Design review of the part built by this model. Coordinates are the model's own, in mm. Face numbers are marked on the shaded views. Give positions to 0.01 mm unless a question says otherwise; leave off trailing zeros. Loops run counter-clockwise (first coordinate to the right, second up) from the corner with the lowest first, then second, coordinate; pieces in that order, holes last. Notation, with made-up numbers: (17.5, -35.75) - (57.5, -35.75) arc R20 cw to (57.5, -20.75) - close; hole circle Ø8 at (-5, 74.25). An arc over 180 degrees is marked (long way). Write each question's results on one line, items separated by ' | '.
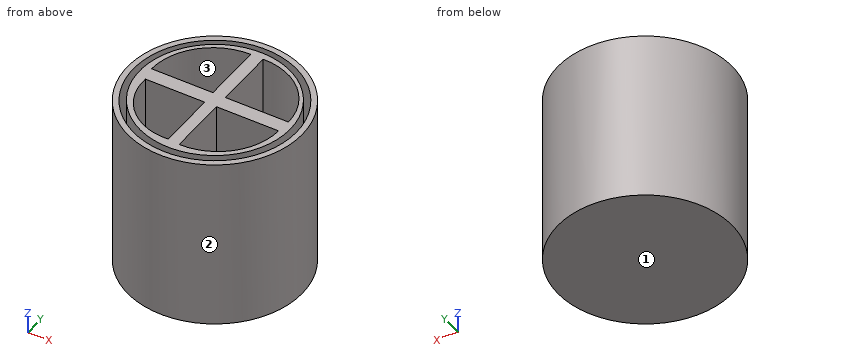
```python
from build123d import *

# Parameters (mm, degrees)
F0_R     = 38.567191
F1_DEPTH = 76.708
F2_T     = -2.54
F3_R     = 33.240041
F4_DEPTH = 74.422
F6_DEPTH = 75.946


with BuildPart() as f1:
    # F0 (on Top) → F1 (new body)
    with BuildSketch(Plane.XY):
        Circle(F0_R)
    extrude(amount=F1_DEPTH)

    # F2
    f2_openings = [f1.faces().sort_by_distance(p)[0] for p in [
        (0, 0, 76.708),
    ]]
    offset(amount=F2_T, openings=f2_openings)

    # F3 (on face) → F4 (join)
    with BuildSketch(Plane.XY.offset(2.54)):
        Circle(F3_R)
    extrude(amount=F4_DEPTH)

    # F5 (on face) → F6 (cut)
    with BuildSketch(Plane.XY.offset(76.962)):
        with BuildLine():
            ThreePointArc((30.418547, 3.318387), (22.14181, 22.611564), (2.580967, 30.234193))
            Line((2.580967, 30.234193), (2.580967, 3.318387))
            Line((2.580967, 3.318387), (30.418547, 3.318387))
        make_face()
        with BuildLine():
            Line((30.049838, -3.134032), (2.580967, -3.134032))
            Line((2.580967, -3.134032), (2.580967, -29.681129))
            ThreePointArc((2.580967, -29.681129), (21.794231, -22.076646), (30.049838, -3.134032))
        make_face()
        with BuildLine():
            Line((-2.949678, 3.318387), (-2.949678, 30.234193))
            ThreePointArc((-2.949678, 30.234193), (-22.011865, 22.326152), (-30.049838, 3.318387))
            Line((-30.049838, 3.318387), (-2.949678, 3.318387))
        make_face()
        with BuildLine():
            Line((-2.580968, -29.128065), (-2.580968, -3.134032))
            Line((-2.580968, -3.134032), (-28.759355, -3.134032))
            ThreePointArc((-28.759355, -3.134032), (-21.580145, -22.082946), (-2.580968, -29.128065))
        make_face()
    extrude(amount=-F6_DEPTH, mode=Mode.SUBTRACT)


solid = f1.part
```
Item 1: We need section D-D on y = -9. Give the boundary of the cut face in (x, z).
Output values:
outline: (-37.5, 0) - (37.5, 0) - (37.5, 76.71) - (34.88, 76.71) - (34.88, 2.54) - (32, 2.54) - (32, 76.96) - (29.29, 76.96) - (29.29, 1.02) - (2.58, 1.02) - (2.58, 76.96) - (-2.58, 76.96) - (-2.58, 1.02) - (-28.43, 1.02) - (-28.43, 76.96) - (-32, 76.96) - (-32, 2.54) - (-34.88, 2.54) - (-34.88, 76.71) - (-37.5, 76.71) - close
Item 2: Wall thickness on probe 1 along Y at (x, z) = (0, 34.5); probe 2 along Y at (x, z) = (-13, 52.5); probe 3 along X at (y, z) = (8, 11.5): over which ranges is each line inside the solid? List them lowest first.
Output values:
probe 1: y = -38.57 to -36.03, -33.24 to 33.24, 36.03 to 38.57 | probe 2: y = -36.31 to -33.6, -30.59 to -27.61, -3.13 to 3.32, 28.26 to 30.59, 33.6 to 36.31 | probe 3: x = -37.73 to -35.13, -32.26 to -29.59, -2.95 to 2.58, 29.97 to 32.26, 35.13 to 37.73
Item 3: We need section A-A on z = 41. Give the boundary of the cut face in (x, y), then the cut area to 3 significant figures.
Output values:
outline: circle Ø77.13 at (0, 0); circle Ø66.48 at (0, 0); hole circle Ø72.05 at (0, 0); hole (-30.05, 3.32) - (-2.95, 3.32) - (-2.95, 30.23) arc R27.22 ccw to start; hole (-28.76, -3.13) arc R24.48 ccw to (-2.58, -29.13) - (-2.58, -3.13) - close; hole (2.58, -29.68) arc R27.08 ccw to (30.05, -3.13) - (2.58, -3.13) - close; hole (2.58, 3.32) - (30.42, 3.32) arc R27.15 ccw to (2.58, 30.23) - close | area: 1,780 mm²
Item 4: We need section B-B on x = 0. Give the boundary of the cut face in (y, z).
Output values:
outline: (-38.57, 0) - (38.57, 0) - (38.57, 76.71) - (36.03, 76.71) - (36.03, 2.54) - (33.24, 2.54) - (33.24, 76.96) - (-33.24, 76.96) - (-33.24, 2.54) - (-36.03, 2.54) - (-36.03, 76.71) - (-38.57, 76.71) - close
Item 5: Draft analysis for pull direction X (two halves, no side actions). For the marked faces 1, 2 and 3, state which applies: +X half, -X half, draft (parallel to the pull), parting line (faces both ways), or undercut.
Output values:
face 1: draft | face 2: parting line | face 3: undercut
Item 6: Clearance check with flat-ended pins moving along their axes: P1, Ø3, axis at x = 18, y = -16, coming from the +Z side; P2, Ø8, axis at x = -10.5, z = 29, coming from the -Y side; P3, Ø12, axis at y = 27.5, z = 26.5, coming from the -X side. State where each tip first meets the part, or that it passes through.
Output values:
P1: stops at z = 1.02 | P2: stops at y = -38.02 | P3: stops at x = -32.02
